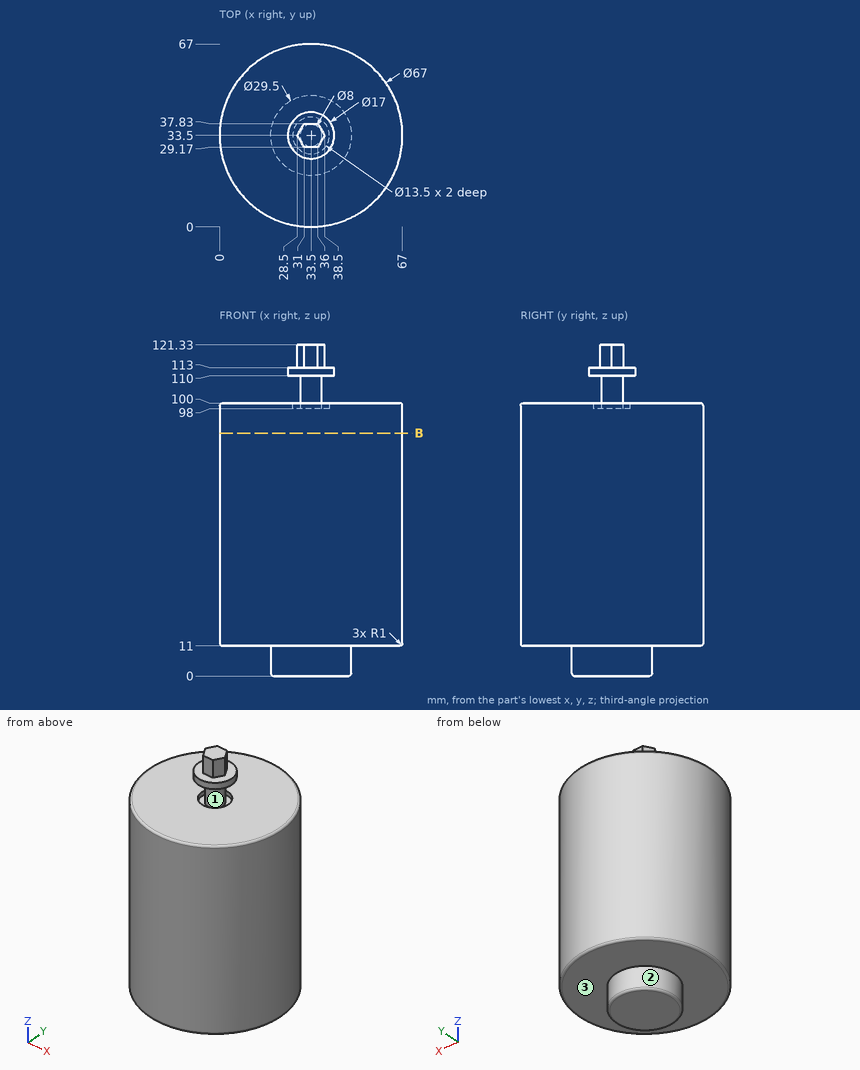
Answer from the drawing. Dimensions are ordinates in mm from the lowest x, y and z of the part. Round coordinates to 2 decimals unless told otherwise and drop trailing zeros. Loops run counter-clockwise (first coordinate to the right, second up) from the corner with the lowest first, then second, coordinate; pieces in that order, holes last.
Q1. Determine the mould class of the marked faces 1, 2 and 3 for opening direction Z: released by +Z, released by -Z, zero draft, split by the parting line, or undercut.
Q2. Consider probe 1 along Y at (x, z) = (33, 99); probe 2 along Z at (x, y) = (11.5, 33). Determine where each line is inside the solid, lowest interval first.
Q3. Each of these flat-tipped pins is pushed along its axis until it touches: pin 1 (8 mm diameter, centred on x = 25, y = 54, fed in from -Z); pin 2 (3 mm diameter, centred on y = 12, z = 45, fed in from +X) (1 decimal); pin 3 (5 mm diameter, centred on y = 40.5, z = 56.5, fed in from -X). Where does it stop, or does it pass through?
Q4. Section B-B on z = 89 is taken. Write down the section's boundary in (x, y).
Output:
1. face 1: undercut
1. face 2: zero draft
1. face 3: released by -Z
2. probe 1: y = 0 to 26.77, 29.53 to 37.47, 40.23 to 67
2. probe 2: z = 11 to 100
3. pin 1: stops at z = 11
3. pin 2: stops at x = 60.4
3. pin 3: stops at x = 0.3
4. outline: circle Ø67 at (33.5, 33.5)
